Design review of the part built by this model. Coordinates are the model's own, in mm. Face numbers are marked on the shaded views. Give positions to 0.01 mm unless a question says otherwise; leave off trailing zeros. Order: outer loops, then holes, each group sorted by start corner. A loop starts at its lowest first (then second) coordinate and runs counter-clockwise, first axis right, second up. Notation, with made-up numbers: M -19.75,70.25 L 0.25,70.25 A26 cw 0.25,85.25 Z; hole C -20.75,46.5 d7. An arc over 180 degrees is marked long. Answer as a JSON object with one key per item and string values.
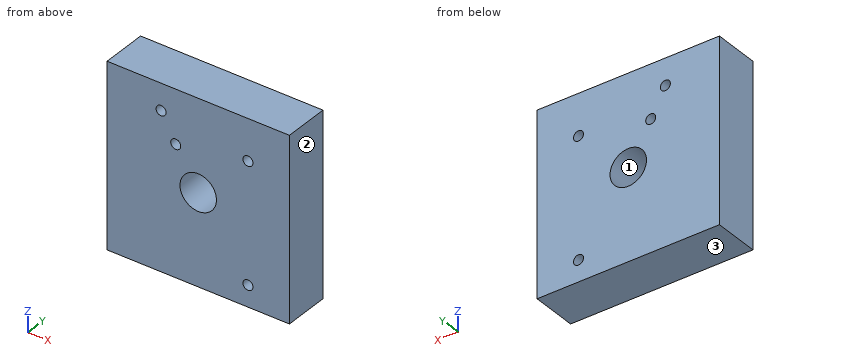
from build123d import *

# Parameters (mm, degrees)
F0_W     = 100
F0_H     = 100
F1_DEPTH = 25
F3_D     = 20
F6_D     = 5.5


with BuildPart() as f1:
    # F0 (on Front) → F1 (new body)
    with BuildSketch(Plane.XZ):
        Rectangle(F0_W, F0_H)
    extrude(amount=F1_DEPTH)

    # F3 (through all)
    with Locations(Plane.XZ.offset(25)):
        with Locations((0, 0)):
            Hole(F3_D / 2)

    # F6 (through all)
    with Locations(Plane.XZ.offset(25)):
        with Locations((27.2540971637, 27.3975413293), (-12.3360659927, 20.7991823554), (-20.3688535839, 35.4303270578), (27.2540971637, -38.2991805673)):
            Hole(F6_D / 2)


solid = f1.part
(1) Draft analysis for pull direction X (two halves, no side actions). For the marked faces 1, 2 and 3, state which applies: +X half, -X half, draft (parallel to the pull), parting line (faces both ways), or undercut.
Checked values:
{"face 1": "undercut", "face 2": "+X half", "face 3": "draft"}
(2) We need section C-C (y = -17.5). Write out the cut boundary in (x, z).
Checked values:
{"outline": "M -50,-50 L 50,-50 L 50,50 L -50,50 Z; hole C -20.37,35.43 d5.5; hole C -12.34,20.8 d5.5; hole C 0,0 d20; hole C 27.25,-38.3 d5.5; hole C 27.25,27.4 d5.5"}
(3) We need section B-B (x = 0). Write out the cut boundary in (y, z).
Checked values:
{"outline": "M -25,-50 L 0,-50 L 0,-10 L -25,-10 Z; M -25,10 L 0,10 L 0,50 L -25,50 Z"}
(4) Insertion check: pin 1 (2 mm diameter, centred on x = -9, z = -19, fed in from +Y); pin 2 (4.5 mm diameter, centred on x = -12.34, z = 20.8, fed in from -Y). Each pin has a flat end and moves straight along its axis. Give the tip position at first contact, or say it passes through.
Checked values:
{"pin 1": "stops at y = 0", "pin 2": "passes through"}
(5) We need section A-A (z = 0). Write out the cut boundary in (x, y).
Checked values:
{"outline": "M -50,-25 L -10,-25 L -10,0 L -50,0 Z; M 10,-25 L 50,-25 L 50,0 L 10,0 Z"}
(6) To check wall thickness, follow L1, parallel to Z at x = 27.5, y = -15; L2, parallel to Z at x = 0, y = -14.5; L3, parallel to Z at x = 28, y = -14. State the ranges of each line that lie inside material, in increasing order. Write a range as from..to.
Checked values:
{"L1": "z = -50..-41.04, -35.56..24.66, 30.14..50", "L2": "z = -50..-10, 10..50", "L3": "z = -50..-40.95, -35.65..24.75, 30.04..50"}
